Model file for the job. Use its own axes, mm. A direction names the side the tool comes from. Coordinates: 2 decimals unless noted, no trailing zeros. Write each loop counter-clockwise with the first axis right and the second up, starting at its lowest first coordinate (ties: lowest second). Pieces come first, ordered by that corner, then holes. Notation, with made-up numbers: M 1.25,82 L 55.25,82 A10 ccw 55.25,96 Z; hole C -23,10.5 d1. An arc over 180 degrees is marked long. One line per question, with ' | ' between items. Start each with the question number.
(1) Tool access for faces 1 (the face through (2, 196.85, -26)), 2 (the face through (30.65, 209, 16)), 3 (the face through (-6.377, 18.98, -20.248)), 4 (the face through (-44.75, 74.71, 27.22)), 5 (the face through (0, 213, 25.65)): list every direction of +Z, -Z, +X, -X, +Y, -Y with a clear straight run to the whole face (end or side of a thin tool).
(2) Two-plate mould, pull along Z, no slides. Class faces 6 (the face through (11, 164.7, 16)), 7 (the face through (-9.2, 203.2, -19.3)), 8 (the face through (-1, 127, 28.825)): +Z half, -Z half, draft (parallel to the pull), parting line (faces both ways), or undercut.
(3) Cut at B-B (y = 105.5). Write the cut outline in (x, z) (3 decimals).
(4) Cut at C-C (x = -3). Write the cut outline in (y, z) (3 decimals), plus the area to 3 significant figures.
(5) Wall check: probe 1 along X at (y, z) = (21, 0); probe 2 along Y at (x, z) = (39.65, 27.8); probe 3 along Y at (x, z) = (19.5, 22). Give the ranges that are in metal, low to high.
(6) Cut at A-A (y = 187.2). Write the cut outline in (x, z) (3 decimals).
(7) Cut at D-D (y = 46). Write the cut outline in (x, z) (3 decimals), plus the area to 3 significant figures.
(8) Flat gauge pins, fed straight in: pin 1 Ø10 at (y, z) = (183.5, 2) entering from -X; pin 2 Ø15.5 at (x, y) = (-39.65, 187.2) entering from -Z; pin 3 Ø8 at (y, z) = (105, 15.5) entering from +X; pin 4 Ø15.5 at (x, y) = (39.65, 46) entering from +Z (3 decimals). Where does each tip first touch, or does it go through?
from build123d import *

# Parameters (mm, degrees)
BOSS_EXTRUDE1_START   = -173.2
BOSS_EXTRUDE1_DEPTH   = 173.2
BOSS_EXTRUDE2_DEPTH   = 3.175
M12_CLEARANCE_HOLE1_D = 13.5
FILLET1_R             = 10
FILLET1_OF_MIRROR1_R  = 10
BOSS_EXTRUDE3_DEPTH   = 6.35
BOSS_EXTRUDE4_DEPTH   = 19.05
CUT_EXTRUDE1_DEPTH    = 238.82533849
FILLET2_R             = 1
FILLET2_OF_MIRROR2_R  = 1


with BuildPart() as part:
    # Sketch12 → Revolve1 (revolve)
    with BuildSketch(Plane.XY, mode=Mode.PRIVATE) as revolve1_sk:
        Polygon((-25.65, 0), (-25.65, 203.2), (-21.22866, 203.2), (-21.22866, 164.7), (-19.177, 164.7), (-19.177, 38.5), (-21.22866, 38.5), (-21.22866, 0), align=None)
    revolve(revolve1_sk.sketch.rotate(Axis((0, 0, 0), (0, 1, 0)), 270), axis=Axis((0, 0, 0), (0, 1, 0)))

    # Sketch14 → Boss-Extrude1 (add)
    with BuildSketch(Plane(origin=(0, 30, 0), x_dir=(-1, 0, 0), z_dir=(0, -1, 0)).offset(BOSS_EXTRUDE1_START)):
        with BuildLine():
            Line((-25.65, 0), (-25.65, -25.65))
            Line((-25.65, -25.65), (1.5e-08, -25.65))
            ThreePointArc((1.5e-08, -25.65), (-18.137288932, -18.137288943), (-25.65, 0))
        make_face()
        with BuildLine():
            ThreePointArc((25.65, 0), (18.137288943, -18.137288932), (1.5e-08, -25.65))
            Line((1.5e-08, -25.65), (25.65, -25.65))
            Line((25.65, -25.65), (25.65, 0))
        make_face()
    extrude(amount=BOSS_EXTRUDE1_DEPTH)

    # Sketch27 → Boss-Extrude2 (add)
    with BuildSketch(Plane.XY.offset(25.65)):
        Polygon((-25.65, 30), (53.65, 30), (53.65, 62), (35.65, 87.706664121), (35.65, 145.493335879), (53.65, 171.2), (53.65, 222.25), (-25.65, 222.25), align=None)
    boss_extrude2 = extrude(amount=BOSS_EXTRUDE2_DEPTH)

    # M12 Clearance Hole1 (through all)
    with Locations(Plane(origin=(0, 0, 25.65), x_dir=(-1, 0, 0), z_dir=(0, 0, -1))):
        with Locations((-39.65, 46), (-39.65, 187.2)):
            m12_clearance_hole1 = Hole(M12_CLEARANCE_HOLE1_D / 2)

    # Fillet1
    fillet1_edges = [part.edges().sort_by_distance(p)[0] for p in [
        (53.65, 222.25, 27.2375),
        (53.65, 30, 27.2375),
        (53.65, 62, 27.2375),
        (35.65, 87.706664121, 27.2375),
        (35.65, 145.493335879, 27.2375),
        (53.65, 171.2, 27.2375),
    ]]
    fillet(fillet1_edges, radius=FILLET1_R)

    # Mirror1: Boss-Extrude2, M12 Clearance Hole1 across plane
    add(boss_extrude2.mirror(Plane(origin=(0, 0, 0), x_dir=(0, 0, 1), z_dir=(1, 0, 0))))
    add(m12_clearance_hole1.mirror(Plane(origin=(0, 0, 0), x_dir=(0, 0, 1), z_dir=(1, 0, 0))), mode=Mode.SUBTRACT)

    # Fillet1 of Mirror1
    fillet1_of_mirror1_edges = [part.edges().sort_by_distance(p)[0] for p in [
        (-53.65, 222.25, 27.2375),
        (-53.65, 30, 27.2375),
        (-53.65, 62, 27.2375),
        (-35.65, 87.706664121, 27.2375),
        (-35.65, 145.493335879, 27.2375),
        (-53.65, 171.2, 27.2375),
    ]]
    fillet(fillet1_of_mirror1_edges, radius=FILLET1_OF_MIRROR1_R)

    # Sketch33 → Boss-Extrude3 (add)
    with BuildSketch(Plane(origin=(0, 203.2, 0), x_dir=(1, 0, 0), z_dir=(0, 1, 0))):
        with BuildLine():
            Line((30.65, -25.65), (30.65, 0))
            ThreePointArc((30.65, 0), (0, 30.65), (-30.65, 0))
            Line((-30.65, 0), (-30.65, -25.65))
            Line((-30.65, -25.65), (-25.65, -25.65))
            Line((-25.65, -25.65), (-25.65, 0))
            ThreePointArc((-25.65, 0), (0, 25.65), (25.65, 0))
            Line((25.65, 0), (25.65, -25.65))
            Line((25.65, -25.65), (30.65, -25.65))
        make_face()
        Polygon((25.65, -25.65), (30.65, -25.65), (30.65, -1.3382079), (25.65, -1.119903186), align=None)
    extrude(amount=-BOSS_EXTRUDE3_DEPTH)

    # Sketch33<3> → Boss-Extrude4 (add)
    with BuildSketch(Plane(origin=(0, 203.2, 0), x_dir=(1, 0, 0), z_dir=(0, 1, 0))):
        Polygon((25.65, -25.65), (30.65, -25.65), (30.65, -1.3382079), (25.65, -1.119903186), align=None)
    boss_extrude4 = extrude(amount=BOSS_EXTRUDE4_DEPTH)

    # Sketch34 → Cut-Extrude1 (cut, symmetric)
    with BuildSketch(Plane(origin=(24.827906129, 0, 1.084009792), x_dir=(0.043619387365336035, 0, -0.9990482215818578), z_dir=(0.9990482215818577, 0, 0.04361938736533603))):
        with BuildLine():
            ThreePointArc((0, 219.9), (-1.643500936, 219.683628997), (-3.175, 219.049261314))
            Line((-3.175, 219.049261314), (0, 213.55))
            Line((0, 213.55), (0, 219.9))
        make_face()
        with BuildLine():
            Line((0, 213.55), (-3.175, 219.049261314))
            ThreePointArc((-3.175, 219.049261314), (-6.35, 213.55), (-3.175, 208.050738686))
            Line((-3.175, 208.050738686), (0, 213.55))
        make_face()
        with BuildLine():
            Line((0, 220.882348419), (-3.175, 219.049261314))
            ThreePointArc((-3.175, 219.049261314), (-1.643500936, 219.683628997), (0, 219.9))
            Line((0, 219.9), (0, 220.882348419))
        make_face()
        with BuildLine():
            Line((0, 207.2), (0, 213.55))
            Line((0, 213.55), (-3.175, 208.050738686))
            ThreePointArc((-3.175, 208.050738686), (-1.643500936, 207.416371003), (0, 207.2))
        make_face()
        with BuildLine():
            ThreePointArc((0, 207.2), (-1.643500936, 207.416371003), (-3.175, 208.050738686))
            Line((-3.175, 208.050738686), (0, 206.217651581))
            Line((0, 206.217651581), (0, 207.2))
        make_face()
    cut_extrude1 = extrude(amount=CUT_EXTRUDE1_DEPTH, both=True, mode=Mode.SUBTRACT)

    # Fillet2
    # the kernel refuses this fillet: 1 mm, written as the material it takes off along each edge
    with BuildSketch(Plane(origin=(33.147620554, 222.25, 1.447256369), x_dir=(-0.04361938736533601, 0, 0.9990482215818578), z_dir=(-0.9990482215818578, 0, -0.043619387365336))) as fillet2_piece_1:
        with BuildLine():
            CenterArc((FILLET2_R, -FILLET2_R), FILLET2_R, 90, 90)
            Line((0, -FILLET2_R), (0, 0))
            Line((0, 0), (FILLET2_R, 0))
        make_face()
    extrude(amount=10.004763426, mode=Mode.SUBTRACT)
    with BuildSketch(Plane(origin=(24.207998101, 220.882348419, 1.056944023), x_dir=(0, 1, 0), z_dir=(0.9990482215818578, 0, 0.043619387365336035))) as fillet2_piece_2:
        with BuildLine():
            CenterArc((FILLET2_R * 0.57735026919, FILLET2_R), FILLET2_R, 210, 60)
            Line((-FILLET2_R * 0.288675134595, FILLET2_R * 0.5), (0, 0))
            Line((0, 0), (FILLET2_R * 0.57735026919, 0))
        make_face()
    extrude(amount=7.891514772, mode=Mode.SUBTRACT)
    with BuildSketch(Plane(origin=(32.092001899, 206.217651581, 1.401167063), x_dir=(-0.03777549755589492, 0.5000000000000023, 0.8652011394955523), z_dir=(-0.9990482215818578, 0, -0.043619387365336035))) as fillet2_piece_3:
        with BuildLine():
            CenterArc((FILLET2_R * 0.57735026919, -FILLET2_R), FILLET2_R, 90, 60)
            Line((-FILLET2_R * 0.288675134595, -FILLET2_R * 0.5), (0, 0))
            Line((0, 0), (FILLET2_R * 0.57735026919, 0))
        make_face()
    extrude(amount=7.891514772, mode=Mode.SUBTRACT)

    # Mirror2: Boss-Extrude4, Cut-Extrude1 across plane
    add(boss_extrude4.mirror(Plane(origin=(0, 0, 0), x_dir=(0, 0, 1), z_dir=(1, 0, 0))))
    add(cut_extrude1.mirror(Plane(origin=(0, 0, 0), x_dir=(0, 0, 1), z_dir=(1, 0, 0))), mode=Mode.SUBTRACT)

    # Fillet2 of Mirror2
    # the kernel refuses this fillet: 1 mm, written as the material it takes off along each edge
    with BuildSketch(Plane(origin=(-33.147620554, 222.25, 1.447256369), x_dir=(0.04361938736533601, 0, 0.9990482215818578), z_dir=(0.9990482215818578, 0, -0.043619387365336))) as fillet2_of_mirror2_piece_1:
        with BuildLine():
            CenterArc((FILLET2_OF_MIRROR2_R, FILLET2_OF_MIRROR2_R), FILLET2_OF_MIRROR2_R, 180, 90)
            Line((0, FILLET2_OF_MIRROR2_R), (0, 0))
            Line((0, 0), (FILLET2_OF_MIRROR2_R, 0))
        make_face()
    extrude(amount=10.004763426, mode=Mode.SUBTRACT)
    with BuildSketch(Plane(origin=(-24.207998101, 220.882348419, 1.056944023), x_dir=(0, 1, 0), z_dir=(-0.9990482215818578, 0, 0.043619387365336035)), Plane(origin=(-32.092001899, 206.217651581, 1.401167063), x_dir=(0, -1, 0), z_dir=(0.9990482215818578, 0, -0.043619387365336035))) as fillet2_of_mirror2_piece_2:
        with BuildLine():
            CenterArc((FILLET2_OF_MIRROR2_R * 0.57735026919, -FILLET2_OF_MIRROR2_R), FILLET2_OF_MIRROR2_R, 90, 60)
            Line((-FILLET2_OF_MIRROR2_R * 0.288675134595, -FILLET2_OF_MIRROR2_R * 0.5), (0, 0))
            Line((0, 0), (FILLET2_OF_MIRROR2_R * 0.57735026919, 0))
        make_face()
    extrude(amount=7.891514772, mode=Mode.SUBTRACT)


solid = part.part
Filled in:
1) face 1: -Z, -Y | face 2: -Z, +X, +Y, -Y | face 3: -Y | face 4: +Z, -Z, -X | face 5: -Z, +Y
2) face 6: undercut | face 7: draft | face 8: +Z half
3) outline: M -35.65,25.65 L -25.65,25.65 L -25.65,0 A25.65 ccw 25.65,0 L 25.65,25.65 L 35.65,25.65 L 35.65,28.825 L -35.65,28.825 Z; hole C 0,0 d38.354
4) outline: M 0,-25.474 L 196.85,-25.474 L 196.85,-30.503 L 203.2,-30.503 L 203.2,-21.016 L 164.7,-21.016 L 164.7,-18.941 L 38.5,-18.941 L 38.5,-21.016 L 0,-21.016 Z; M 0,21.016 L 38.5,21.016 L 38.5,18.941 L 164.7,18.941 L 164.7,21.016 L 203.2,21.016 L 203.2,25.65 L 222.25,25.65 L 222.25,28.825 L 30,28.825 L 30,25.474 L 0,25.474 Z | area: 3,010 mm²
5) probe 1: -25.65 to -21.23, 21.23 to 25.65 | probe 2: 30 to 39.25, 52.75 to 81.99, 151.21 to 180.45, 193.95 to 222.25 | probe 3: 30 to 203.2
6) outline: M -53.65,25.65 L -46.4,25.65 L -46.4,28.825 L -53.65,28.825 Z; M -32.9,25.65 L -25.65,25.65 L -25.65,0 A25.65 ccw 25.65,0 L 25.65,25.65 L 32.9,25.65 L 32.9,28.825 L -32.9,28.825 Z; M 46.4,25.65 L 53.65,25.65 L 53.65,28.825 L 46.4,28.825 Z; hole C 0,0 d42.457
7) outline: M -53.65,25.65 L -46.4,25.65 L -46.4,28.825 L -53.65,28.825 Z; M -32.9,25.65 L -25.65,25.65 L -25.65,0 A25.65 ccw 25.65,0 L 25.65,25.65 L 32.9,25.65 L 32.9,28.825 L -32.9,28.825 Z; M 46.4,25.65 L 53.65,25.65 L 53.65,28.825 L 46.4,28.825 Z; hole C 0,0 d38.354 | area: 1,450 mm²
8) pin 1: x = -25.65 | pin 2: z = 25.65 | pin 3: x = 25.65 | pin 4: z = 28.825
